Can you work these out from the model? Positions are in its coordinate system, mm. Face numbers are marked on the shaded views. A direction names the side the tool comes from. Give positions to 0.01 mm unless a question says otherwise; leave off trailing zeros. Write each loop counter-clockwise with the first axis right and the second up, starting at its lowest first coordinate (ties: lowest second). Pieces come first, ordered by that corner, then holes. Notation, with made-up numbers: M 88.5,-32.75 L 115.5,-32.75 A18 ccw 115.5,-9.75 Z; hole C 0.25,-2 d5. An arc over 180 degrees is marked long. Write each question's results on one line, items separated by ' | '.
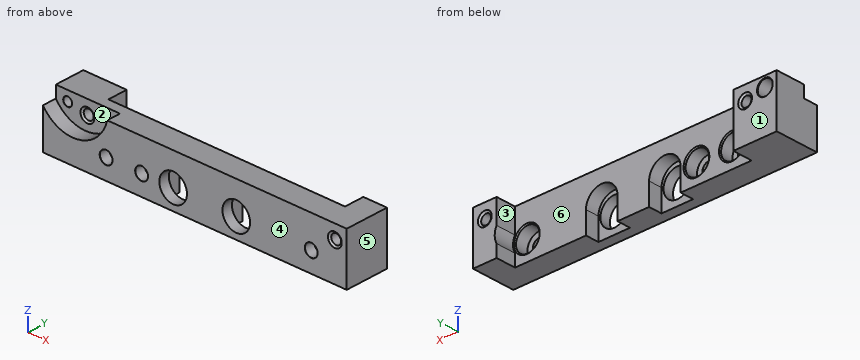
from build123d import *

# Parameters (mm, degrees)
SKETCH_1_W                 = 13
SKETCH_1_H                 = 11
EXTRUDE_1_DEPTH            = 77
SKETCH_2_W                 = 60
SKETCH_2_H                 = 5
CUT_EXTRUDE_1_DEPTH        = 79.860636569
CUT_EXTRUDE_2_DEPTH        = 5
HOLE_WIZARD_M31_AT_2_COUNT = 2
HOLE_WIZARD_M31_AT_2_PITCH = 52
HOLE_WIZARD_M31_AT_3_COUNT = 2
HOLE_WIZARD_M31_AT_3_PITCH = 9
CUT_EXTRUDE_3_DEPTH        = 3.5
CUT_EXTRUDE_5_DEPTH        = 3.4
SKETCH_12_R                = 3.5
CUT_EXTRUDE_6_DEPTH        = 10


# Read off the part's stored shape, not the designer's step: Отверстие обработанное метчиком M32
with BuildPart() as part:
    # Эскиз1 → Бобышка-Вытянуть1 (new body)
    with BuildSketch(Plane(origin=(0, 0, 0), x_dir=(0, 0, -1), z_dir=(1, 0, 0))):
        with Locations((6.5, 5.5)):
            Rectangle(SKETCH_1_W, SKETCH_1_H)
    extrude(amount=EXTRUDE_1_DEPTH)

    # Эскиз2 → Вырез-Вытянуть1 (cut, through all)
    with BuildSketch(Plane.XY):
        with Locations((41, 8.5)):
            Rectangle(SKETCH_2_W, SKETCH_2_H)
    extrude(amount=-CUT_EXTRUDE_1_DEPTH, mode=Mode.SUBTRACT)

    # Эскиз5 → Вырез-Вытянуть2 (cut)
    with BuildSketch(Plane(origin=(0, 11, 0), x_dir=(1, 0, 0), z_dir=(0, 1, 0))):
        with BuildLine():
            ThreePointArc((71, 6.063508327), (71.5, 8), (71, 9.936491673))
            Line((71, 9.936491673), (71, 6.063508327))
        make_face()
    extrude(amount=-CUT_EXTRUDE_2_DEPTH, mode=Mode.SUBTRACT)

    # Эскиз3 → Цековка для винта с внутренним шестигранником M31 (revolve, cut)
    with BuildSketch(Plane(origin=(16, 6, -8), x_dir=(0, 0, 1), z_dir=(1, 0, 0))):
        Polygon((0, 0), (0, 6), (1.625, 6), (1.6, 5.975), (1.6, 3.425), (1.625, 3.4), (3, 3.4), (3, 0.275), (3.275, 0), align=None)
    hole_wizard_m31 = revolve(axis=Axis((16, 12.35, -8), (0, -1, 0)), mode=Mode.SUBTRACT)

    # Цековка для винта с внутренним шестигранником M31 at 2: Цековка для винта с внутренним шестигранником M31 ×2
    with Locations(*[(i * HOLE_WIZARD_M31_AT_2_PITCH, 0, 0) for i in range(1, HOLE_WIZARD_M31_AT_2_COUNT)]):
        add(hole_wizard_m31, mode=Mode.SUBTRACT)

    # Цековка для винта с внутренним шестигранником M31 at 3: Цековка для винта с внутренним шестигранником M31 ×2
    with Locations(*[(i * HOLE_WIZARD_M31_AT_3_PITCH, 0, 0) for i in range(1, HOLE_WIZARD_M31_AT_3_COUNT)]):
        add(hole_wizard_m31, mode=Mode.SUBTRACT)

    # Эскиз8 → Вырез-Вытянуть3 (cut)
    with BuildSketch(Plane.XZ):
        with BuildLine():
            ThreePointArc((0, -2.974937186), (9.118315903, -6.853307497), (16.274964387, 0))
            Line((16.274964387, 0), (0, 0))
            Line((0, 0), (0, -2.974937186))
        make_face()
    extrude(amount=-CUT_EXTRUDE_3_DEPTH, mode=Mode.SUBTRACT)

    # Эскиз9 → Вырез-Вытянуть5 (cut)
    with BuildSketch(Plane.XZ.offset(-6)):
        with BuildLine():
            ThreePointArc((37, -7.5), (33, -3.5), (29, -7.5))
            Line((29, -7.5), (29, -13))
            Line((29, -13), (37, -13))
            Line((37, -13), (37, -7.5))
        make_face()
        with BuildLine():
            Line((45, -7.5), (45, -13))
            Line((45, -13), (53, -13))
            Line((53, -13), (53, -7.5))
            ThreePointArc((53, -7.5), (49, -3.5), (45, -7.5))
        make_face()
    extrude(amount=CUT_EXTRUDE_5_DEPTH, mode=Mode.SUBTRACT)

    # Отверстие обработанное метчиком M32 outline → Отверстие обработанное метчиком M32 (revolve, cut)
    with BuildSketch(Plane(origin=(74, 0, -3.5), x_dir=(1, 0, 0), z_dir=(0, 0, 1))):
        Polygon((0, 0), (1.75, 0), (1.25, 0.350103769), (1.25, 10.649896231), (1.75, 11), (0, 11), align=None)
    revolve(axis=Axis((74, 0, -3.5), (0, 1, 0)), mode=Mode.SUBTRACT)

    # Hole Wizard M32 2 outline → Hole Wizard M32 2 (revolve, cut)
    with BuildSketch(Plane(origin=(8, 0, -3.5), x_dir=(1, 0, 0), z_dir=(0, 0, 1))):
        Polygon((0, 3.5), (1.75, 3.5), (1.25, 3.850103769), (1.25, 10.649896231), (1.75, 11), (0, 11), align=None)
    revolve(axis=Axis((8, 0, -3.5), (0, 1, 0)), mode=Mode.SUBTRACT)

    # Эскиз10 → Цековка для винта с внутренним шестигранником M21 (revolve, cut)
    with BuildSketch(Plane(origin=(3, 11, -2.5), x_dir=(0, 0, 1), z_dir=(1, 0, 0))):
        Polygon((0, 0), (0, 7.5), (1.125, 7.5), (1.1, 7.475), (1.1, 3.525), (1.125, 3.5), (1.9, 3.5), (1.9, 0.1), (2, 0), align=None)
    revolve(axis=Axis((3, 17.35, -2.5), (0, -1, 0)), mode=Mode.SUBTRACT)

    # Эскиз12 → Вырез-Вытянуть6 (cut)
    with BuildSketch(Plane(origin=(0, 6, 0), x_dir=(1, 0, 0), z_dir=(0, 1, 0))):
        with Locations(Location((33, 8, 0), (0, 0, 270))):
            Circle(SKETCH_12_R)
        with Locations(Location((49, 8, 0), (0, 0, 270))):
            Circle(SKETCH_12_R)
    extrude(amount=-CUT_EXTRUDE_6_DEPTH, mode=Mode.SUBTRACT)


solid = part.part
Item 1: I want a section at A-A, the plane y = 9. Please give me the cut outline in (x, z).
Geometry says:
outline: M 0,-13 L 11,-13 L 11,0 L 0,0 Z; M 71,-13 L 77,-13 L 77,0 L 71,0 L 71,-6.06 A4 cw 71,-9.94 Z; hole C 3,-2.5 d3.8; hole C 8,-3.5 d2.5; hole C 74,-3.5 d2.5
Item 2: Thinking about a two-plate mould opening in X: for the marked faces 4, 5 and 6, which applies, +X half, -X half, draft (parallel to the pull), parting line (faces both ways), or undercut?
Geometry says:
face 4: draft | face 5: +X half | face 6: undercut
Item 3: I want a section at B-B, the plane x = 68. Please give me the cut outline in (y, z) (3 decimals).
Geometry says:
outline: M 0,-13 L 6,-13 L 6,-11.275 L 5.725,-11 L 2.6,-11 L 2.6,-9.625 L 2.575,-9.6 L 0.025,-9.6 L 0,-9.625 Z; M 0,-6.375 L 0.025,-6.4 L 2.575,-6.4 L 2.6,-6.375 L 2.6,-5 L 5.725,-5 L 6,-4.725 L 6,0 L 0,0 Z
Item 4: If I drill on line 1 (X direction, y = 1.8, z = -8); line 2 (Z direction, x = 74, y = 5.75); line 3 (X direction, y = 5.75, z = -10), over which ranges is the centre line in solid material (lowest first)? Write a range as from..to.
Geometry says:
line 1: x = 0..14.4, 17.6..23.4, 26.6..29.5, 36.5..45.5, 52.5..66.4, 69.6..77 | line 2: z = -13..-4.75, -2.25..0 | line 3: x = 0..13.73, 18.27..22.73, 27.27..29, 37..45, 53..65.73, 70.27..77
Item 5: For the marked faces 1, 2 and 3, which set-ups out of +Z, -Z, +X, -X, +Y, -Y let a thin tool reach every point of the face, with its end or its side?
Geometry says:
face 1: +Z, -Z, +X, -X, +Y | face 2: +Z, -Y | face 3: +Z, -Z, +Y
Item 6: I want a section at D-D, the plane x = 49. Please give me the cut outline in (y, z).
Geometry says:
outline: M 0,-13 L 2.6,-13 L 2.6,-11.5 L 0,-11.5 Z; M 0,-4.5 L 2.6,-4.5 L 2.6,-3.5 L 6,-3.5 L 6,0 L 0,0 Z
Item 7: I want a section at C-C, the plane y = 5. Please give me the cut outline in (x, z), and give its area (3 significant figures).
Geometry says:
outline: M 0,-13 L 29,-13 L 29,-7.5 A4 cw 37,-7.5 L 37,-13 L 45,-13 L 45,-7.5 A4 cw 53,-7.5 L 53,-13 L 77,-13 L 77,0 L 0,0 Z; hole C 3,-2.5 d2.2; hole C 8,-3.5 d2.5; hole C 16,-8 d6; hole C 25,-8 d6; hole C 68,-8 d6; hole C 74,-3.5 d2.5 | area: 764 mm2
Item 8: I'm going to push flat-ended pins straight in: pin 1 (3 mm diameter, centred on x = 74, z = -3.5, fed in from +Y); pin 2 (2 mm diameter, centred on x = 9, z = -5, fed in from -Y); pin 3 (5 mm diameter, centred on x = 68, z = -8, fed in from +Y); pin 4 (4 mm diameter, centred on x = 29.5, z = -4, fed in from -Y). Where does each tip first touch, or does it pass through?
Geometry says:
pin 1: stops at y = 10.82 | pin 2: stops at y = 3.5 | pin 3: stops at y = 2.6 | pin 4: stops at y = 0
